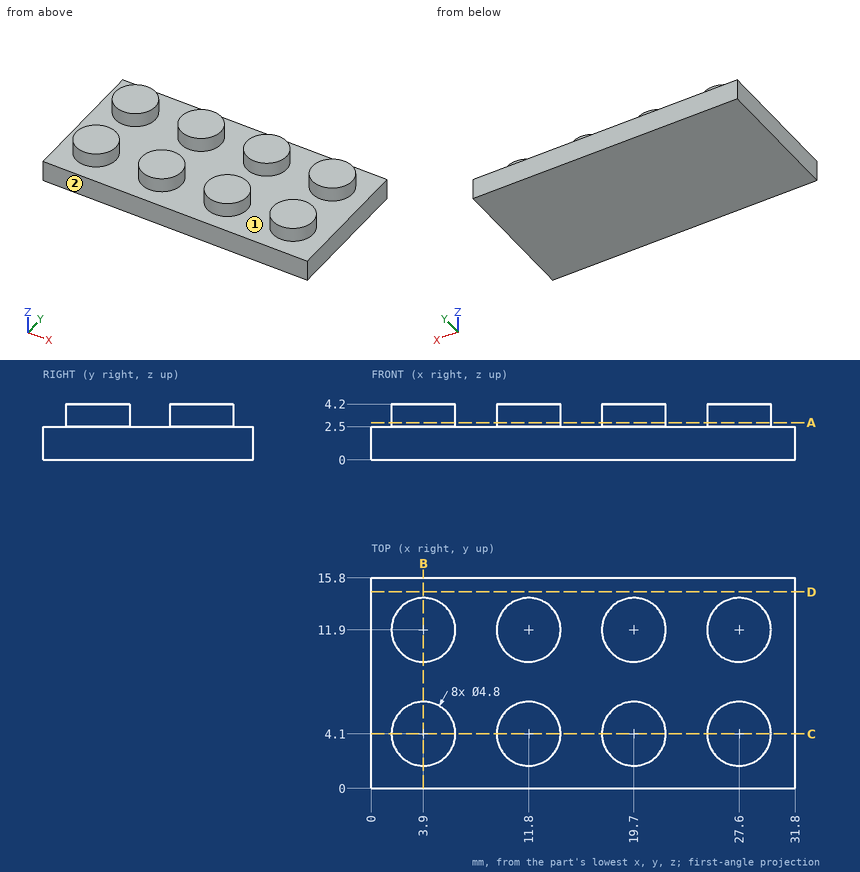
Input: dimensioned drawing with shaded views. Units: mm. Origin: part minimum x, y, z. Coordinates: 2 decimals unless noted, no trailing zeros. Loops run counter-clockwise (first coordinate to the right, second up) from the corner with the lowest first, then second, coordinate; pieces in that order, holes last. Notation, with made-up numbers: M -12.75,14 L 30.25,14 A32 cw 30.25,44 Z; hole C 13.25,-7 d2. An arc over 180 degrees is marked long. One line per item, written item: value. Start each with the question number.
1) Pin query (flat end, axial travel): P1, Ø1, axis at y = 11.5, z = 1, coming from the -X side. Return the tip coordinate at first contact, or that it passes through.
2) Cut plane D-D (y = 14.75). Return loops of the section in (x, z).
3) Draft query along X for the marked faces 1 and 2. Return one class per face: released by +X, released by -X, zero draft, split by the parting line, or undercut.
4) Cut plane A-A (z = 2.8). Return loops of the section in (x, y), then the cut area to 3 significant figures.
5) Cut plane B-B (x = 3.9). Return loops of the section in (y, z), then the cut area to 3 significant figures.
6) Material intervals for L1, parallel to X at y = 10.25, z = 3.9; L2, parallel to X at y = 6, z = 3.45; L3, parallel to Z at x = 23, y = 11.5, sorted ascending. Write a range as from..to.
7) Cut plane C-C (y = 4.1). Return loops of the section in (x, z).
Evaluation:
1. P1: x = 0
2. outline: M 0,0 L 31.8,0 L 31.8,2.5 L 0,2.5 Z
3. face 1: undercut
3. face 2: zero draft
4. outline: C 3.9,4.1 d4.8; C 3.9,11.9 d4.8; C 11.8,4.1 d4.8; C 11.8,11.9 d4.8; C 19.7,4.1 d4.8; C 19.7,11.9 d4.8; C 27.6,4.1 d4.8; C 27.6,11.9 d4.8
4. area: 145 mm^2
5. outline: M 0,0 L 15.8,0 L 15.8,2.5 L 14.3,2.5 L 14.3,4.2 L 9.5,4.2 L 9.5,2.5 L 6.5,2.5 L 6.5,4.2 L 1.7,4.2 L 1.7,2.5 L 0,2.5 Z
5. area: 55.8 mm^2
6. L1: 2.16..5.64, 10.06..13.54, 17.96..21.44, 25.86..29.34
6. L2: 2.43..5.37, 10.33..13.27, 18.23..21.17, 26.13..29.07
6. L3: 0..2.5
7. outline: M 0,0 L 31.8,0 L 31.8,2.5 L 30,2.5 L 30,4.2 L 25.2,4.2 L 25.2,2.5 L 22.1,2.5 L 22.1,4.2 L 17.3,4.2 L 17.3,2.5 L 14.2,2.5 L 14.2,4.2 L 9.4,4.2 L 9.4,2.5 L 6.3,2.5 L 6.3,4.2 L 1.5,4.2 L 1.5,2.5 L 0,2.5 Z
